from build123d import *

# Parameters (mm, degrees)
EXTRUDE_1_DEPTH      = 1
SKETCH_2_R           = 1
EXTRUDE_3_DEPTH      = 1.5
EXTRUDE_3_DEPTH_BACK = 1.5
EXTRUDE_4_DEPTH      = 30
SKETCH_4_R           = 1.25
CUT_EXTRUDE_1_DEPTH  = 4.330127


with BuildPart() as part:
    # 스케치1 → 보스-돌출1 (new body)
    with BuildSketch(Plane.XY):
        Polygon((0, 4), (-3.464101615, 2), (-3.464101615, -2), (0, -4), (3.464101615, -2), (3.464101615, 2), align=None)
    extrude(amount=EXTRUDE_1_DEPTH)

    # 스케치2 → 보스-돌출3 (add, two sides)
    with BuildSketch(Plane(origin=(0, 0, 0), x_dir=(1, 0, 0), z_dir=(0, 1, 0))) as extrude_3_sk:
        with BuildLine():
            Line((-3.464101615, -1), (3.464101615, -1))
            Line((3.464101615, -1), (3.464101615, -5))
            ThreePointArc((3.464101615, -5), (0, -8.464101615), (-3.464101615, -5))
            Line((-3.464101615, -5), (-3.464101615, -1))
        make_face()
        with Locations((0, -5)):
            Circle(SKETCH_2_R, mode=Mode.SUBTRACT)
    extrude(amount=EXTRUDE_3_DEPTH)
    extrude(extrude_3_sk.sketch, amount=-EXTRUDE_3_DEPTH_BACK)

    # 스케치3 → 보스-돌출4 (add)
    with BuildSketch(Plane(origin=(0, 0, 0), x_dir=(-1, 0, 0), z_dir=(0, 0, -1))):
        Polygon((0, 2.5), (-2.165063509, 1.25), (-2.165063509, -1.25), (0, -2.5), (2.165063509, -1.25), (2.165063509, 1.25), align=None)
    extrude(amount=EXTRUDE_4_DEPTH)

    # 스케치4 → 컷-돌출1 (cut)
    with BuildSketch(Plane.ZY.offset(2.165063509)):
        with Locations((-26.75, 0)):
            Circle(SKETCH_4_R)
    extrude(amount=-CUT_EXTRUDE_1_DEPTH, mode=Mode.SUBTRACT)


solid = part.part
Read the model definition and answer for the solid it produces. Units are mm, in the model's axes. A direction names the side the tool comes from. Round coordinates to 2 decimals unless told otherwise and drop trailing zeros. Write each loop counter-clockwise with the first axis right and the second up, starting at its lowest first coordinate (ties: lowest second). Pieces come first, ordered by that corner, then holes.
1. Determine the mould class of faces 1 (the face through (-0.03, -0.479, -25.595)), 2 (the face through (-1.756, -2.986, 0.493)), 3 (the face through (-2, -2, 0)), 4 (the face through (-1.098, 1.866, -14.79)) for opening direction Y: pulls with the +Y half, pulls with the -Y half, needs draft (parallel to the pull), parting line crosses it, or undercut.
2. Straight lines are drawn through the part: L1, parallel to Z at x = 0, y = 0.4; L2, parallel to X at y = 0.75, z = 5; L3, parallel to Z at x = 0, y = 1.1. For each, find the intervals that lie inside material, in ascending order.
3. The part is cut by section B-B, the plane z = -23.5. Determine the outline of the cut face in (x, y).
4. The part is cut by section C-C, the plane x = -2.75. Determine the outline of the cut face in (y, z), then the cut area to 3 significant figures.
5. Which of the six approach directions +Z, -Z, +X, -X, +Y, -Y give full straight-line access (tool end or side, diameter ignored) to faces 5 (the face through (0, -2, 1)), 6 (the face through (-2.165, 0, -13)), 7 (the face through (1.098, -1.866, -14.79)), 8 (the face through (-1.07, -1.88, -14.79)), 9 (the face through (0.05, 1.5, 3.85))?
6. The part is cut by section A-A, the plane y = -0.5. Determine the outline of the cut face in (x, z).
7. Given pin 1 Ø4 at (y, z) = (0, -26.75) entering from -X; pin 2 Ø2 at (y, z) = (0.5, -29) entering from +X; pin 3 Ø0.8 at (x, y) = (1, 2.5) entering from +Z, each flat-ended and moving along its own axis, determine where each tip first touches the part or whether it passes through.
8. The part is cut by section D-D, the plane x = 1.75. Determine the outline of the cut face in (y, z).
Values:
1. face 1: undercut
1. face 2: pulls with the -Y half
1. face 3: needs draft
1. face 4: pulls with the +Y half
2. L1: z = -30 to -27.93, -25.57 to 4, 6 to 8.46
2. L2: x = -3.46 to -1, 1 to 3.46
2. L3: z = -30 to -27.34, -26.16 to 4, 6 to 8.46
3. outline: (-2.17, -1.25) - (0, -2.5) - (2.17, -1.25) - (2.17, 1.25) - (0, 2.5) - (-2.17, 1.25) - close
4. outline: (-2.41, 0) - (2.41, 0) - (2.41, 1) - (1.5, 1) - (1.5, 7.11) - (-1.5, 7.11) - (-1.5, 1) - (-2.41, 1) - close
4. area: 23.1 mm2
5. face 5: +Z, +X, -X, -Y
5. face 6: -Z, -X, +Y, -Y
5. face 7: -Z, +X, -Y
5. face 8: -Z, -X, -Y
5. face 9: +Z, +X, -X, +Y
6. outline: (-3.46, 0) - (-2.17, 0) - (-2.17, -25.6) - (2.17, -25.6) - (2.17, 0) - (3.46, 0) - (3.46, 5) arc R3.46 ccw to (-3.46, 5) - close; (-2.17, -30) - (2.17, -30) - (2.17, -27.9) - (-2.17, -27.9) - close; hole circle Ø2 at (0, 5)
7. pin 1: stops at x = -2.17
7. pin 2: stops at x = 2.17
7. pin 3: stops at z = 1
8. outline: (-2.99, 0) - (-1.49, 0) - (-1.49, -30) - (1.49, -30) - (1.49, 0) - (2.99, 0) - (2.99, 1) - (1.5, 1) - (1.5, 7.99) - (-1.5, 7.99) - (-1.5, 1) - (-2.99, 1) - close; hole circle Ø2.5 at (0, -26.75)
